The model under review builds one solid part; all positions refer to its coordinate system, in mm. Round coordinates to 2 decimals unless told otherwise and drop trailing zeros. Write each loop counter-clockwise with the first axis right and the second up, starting at its lowest first coordinate (ties: lowest second). Pieces come first, ordered by that corner, then holes. Notation, with made-up numbers: (18.25, -25) -> (77.25, -25) arc R10 ccw to (77.25, -19) -> close; hole circle Ø10 at (51.25, -39). An arc over 180 degrees is marked (long way). Answer as a JSON object with one key per item and string values. Group by question number.
1) We need section C-C, the plane y = 0.6. Write out the cut boundary in (x, z), then the cut area to 3 significant figures.
2) We need section A-A, the plane z = 0. Write out the cut boundary in (x, y), then the cut area to 3 significant figures.
3) To check wall thickness, follow probe 1 along Y at (x, z) = (-43, -1.5); probe 2 along X at (y, z) = (1.75, -0.85). State the ranges of each line that lie inside material, in increasing order. Write a range as [from, to].
4) Insertion check: pin 1 Ø2 at (x, z) = (-16, 0.5) entering from +Y; pin 2 Ø1 at (x, y) = (-14, 1) entering from -Z; pin 3 Ø0.6 at (y, z) = (2, 0) entering from -X. Each pin has a flat end and moves straight along its axis. Give the tip position at first contact, or say it passes through.
5) We need section B-B, the plane x = 21. Write out the cut boundary in (y, z), then the cut area to 3 significant figures.
6) We need section D-D, the plane x = -61. Write out the cut boundary in (y, z).
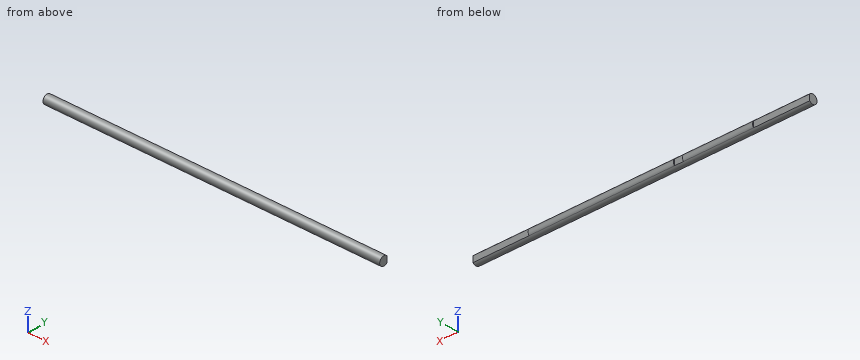
from build123d import *

# Parameters (mm, degrees)
BOSS_EXTRUDE1_DEPTH     = 75
SKETCH2_R               = 2
BOSS_EXTRUDE2_DEPTH     = 50
SKETCH3_W               = 4
SKETCH3_H               = 0.5
CUT_EXTRUDE1_DEPTH      = 3
CUT_EXTRUDE1_DEPTH_BACK = 3


with BuildPart() as part:
    # Sketch1 → Boss-Extrude1 (new body, symmetric)
    with BuildSketch(Plane(origin=(0, 0, 0), x_dir=(0, 0, -1), z_dir=(1, 0, 0))):
        with BuildLine():
            Line((-1.322875656, 1.5), (1.322875656, 1.5))
            ThreePointArc((1.322875656, 1.5), (0, -2), (-1.322875656, 1.5))
        make_face()
    extrude(amount=BOSS_EXTRUDE1_DEPTH, both=True)

    # Sketch2 → Boss-Extrude2 (add, symmetric)
    with BuildSketch(Plane(origin=(0, 0, 0), x_dir=(0, 0, -1), z_dir=(1, 0, 0))):
        Circle(SKETCH2_R)
    extrude(amount=BOSS_EXTRUDE2_DEPTH, both=True)

    # Sketch3 → Cut-Extrude1 (cut, two sides)
    with BuildSketch(Plane.XY) as cut_extrude1_sk:
        with Locations((-16.76, 1.75)):
            Rectangle(SKETCH3_W, SKETCH3_H)
    extrude(amount=CUT_EXTRUDE1_DEPTH, mode=Mode.SUBTRACT)
    extrude(cut_extrude1_sk.sketch, amount=-CUT_EXTRUDE1_DEPTH_BACK, mode=Mode.SUBTRACT)


solid = part.part
Here are the results:
{
 "1": {"outline": "(-75, -1.91) -> (75, -1.91) -> (75, 1.91) -> (-75, 1.91) -> close", "area": "572 mm^2"},
 "2": {"outline": "(-75, -2) -> (75, -2) -> (75, 1.5) -> (50, 1.5) -> (50, 2) -> (-14.76, 2) -> (-14.76, 1.5) -> (-18.76, 1.5) -> (-18.76, 2) -> (-50, 2) -> (-50, 1.5) -> (-75, 1.5) -> close", "area": "573 mm^2"},
 "3": {"probe 1": "y = [-1.32, 1.32]", "probe 2": "x = [-50, -18.76], [-14.76, 50]"},
 "4": {"pin 1": "stops at y = 1.5", "pin 2": "stops at z = -1.94", "pin 3": "stops at x = -50"},
 "5": {"outline": "circle Ø4 at (0, 0)", "area": "12.6 mm^2"},
 "6": {"outline": "(1.5, -1.32) -> (1.5, 1.32) arc R2 ccw (long way) to start"}
}
